Model file for the job. Use its own axes, mm. A direction names the side the tool comes from. Coordinates: 2 decimals unless noted, no trailing zeros. Write each loop counter-clockwise with the first axis right and the second up, starting at its lowest first coordinate (ties: lowest second). Pieces come first, ordered by that corner, then holes. Notation, with made-up numbers: M -32,81 L -5,81 A11 ccw -5,96 Z; hole C 14.5,88.5 d11. An arc over 180 degrees is marked long. One line per question, with ' | ' between items. Start each with the question number.
(1) Flat gauge pins, fed straight in: pin 1 Ø9 at (x, z) = (-27, 10) entering from -Y; pin 2 Ø1.5 at (x, z) = (39.5, 25.5) entering from +Y; pin 3 Ø10 at (x, z) = (33.5, 8) entering from +Y. Where does each tip first touch, or does it go through?
(2) Cut at B-B (x = 40.5). Write the cut outline in (y, z), plus the area to 3 significant figures.
(3) Cut at A-A (y = -12.5). Write the cut outline in (x, z).
(4) Tool access for faces 1 (the face through (27.825, -41, 15)), 2 (the face through (-20, 34.557, 15)), 3 (the face through (27, -21, 30)): list every direction of +Z, -Z, +X, -X, +Y, -Y with a clear straight run to the whole face (end or side of a thin tool).
(5) Wall check: probe 1 along Y at (x, z) = (31.5, 18); probe 2 along X at (y, z) = (-53.5, 2.5); probe 3 along Y at (x, z) = (-13, 20). Give the ranges that are in metal, low to high.
from build123d import *

# Parameters (mm, degrees)
BOSS_EXTRUDE1_DEPTH = 30


with BuildPart() as part:
    # Sketch1 → Boss-Extrude1 (new body)
    with BuildSketch(Plane.XY):
        with BuildLine():
            Line((-40, 38.556946986), (0, 38.556946986))
            add(Edge.make_bspline(
                [(0, 38.556946986), (25.885340012, 28.023752492), (27.824600918, 0.131180898)],
                knots=[0, 0, 0, 1, 1, 1], degree=2))
            Line((27.824600918, 0.131180898), (27.824600918, -82.868819102))
            ThreePointArc((27.824600918, -82.868819102), (28.703280574, -84.990139445), (30.824600918, -85.868819102))
            Line((30.824600918, -85.868819102), (62.541306618, -85.868819102))
            Line((62.541306618, -85.868819102), (62.541306618, -89.868819102))
            Line((62.541306618, -89.868819102), (27.824600918, -89.868819102))
            Line((27.824600918, -89.868819102), (26.824600918, -89.868819102))
            ThreePointArc((26.824600918, -89.868819102), (24.703280574, -88.990139445), (23.824600918, -86.868819102))
            Line((23.824600918, -86.868819102), (23.824600918, -0.01001344))
            add(Edge.make_bspline(
                [(-0.796307781, 34.556946986), (-0.313071462, 34.352718519), (0.65471267, 33.927572325), (2.509371581, 33.047404589), (4.716407797, 31.874992229), (7.176880305, 30.35963937), (10.215802607, 28.194209311), (13.569039872, 25.21811291), (16.917231379, 21.206114841), (19.621581596, 16.724458997), (21.351620726, 12.565197335), (22.419479521, 8.964412879), (23.060246931, 6.124694742), (23.459149076, 3.637055451), (23.695469018, 1.580241662), (23.786657543, 0.517816431), (23.824600918, -0.01001344)],
                knots=[0.014797718, 0.014797718, 0.014797718, 0.014797718, 0.045503656, 0.076209593, 0.137621468, 0.199033343, 0.260445218, 0.383268968, 0.506092718, 0.628916468, 0.751740218, 0.813152093, 0.874563968, 0.935975843, 0.966681781, 0.997387718, 0.997387718, 0.997387718, 0.997387718], degree=3))
            Line((-0.796307781, 34.556946986), (-40, 34.556946986))
            Line((-40, 34.556946986), (-40, 38.556946986))
        make_face()
    extrude(amount=BOSS_EXTRUDE1_DEPTH)


solid = part.part
Filled in:
1) pin 1: y = 34.56 | pin 2: y = -85.87 | pin 3: y = -84.77
2) outline: M -89.87,0 L -85.87,0 L -85.87,30 L -89.87,30 Z | area: 120 mm²
3) outline: M 23.82,0 L 27.82,0 L 27.82,30 L 23.82,30 Z
4) face 1: +Z, -Z, +X, +Y | face 2: +Z, -Z, -X, -Y | face 3: +Z, +X, -X, +Y, -Y
5) probe 1: -89.87 to -85.87 | probe 2: 23.82 to 27.82 | probe 3: 34.56 to 38.56
